Input: part model. Units: mm. Frame: model coordinates. Coordinates: 2 decimals unless noted, no trailing zeros. Write each loop counter-clockwise with the first axis right and the second up, starting at its lowest first coordinate (ties: lowest second). Pieces come first, ordered by that corner, then holes. Notation, with made-up numbers: (17, 28) - (53, 28) arc R20 cw to (53, 60) - close; hole circle Ø11 at (46, 16.5). An arc over 180 degrees is marked (long way). Use CSV: the item, a comma, the result in double quotes.
```python
from build123d import *

# Parameters (mm, degrees)
SKETCH3_R           = 38.1
BOSS_EXTRUDE2_DEPTH = 50.8
SKETCH4_R           = 19.05
FILLET1_R           = 12.7
SKETCH5_R           = 19.05


with BuildPart() as part:
    # Sketch3 → Boss-Extrude2 (new body)
    with BuildSketch(Plane.XY):
        with Locations((0, 177.8)):
            Circle(SKETCH3_R)
    extrude(amount=BOSS_EXTRUDE2_DEPTH)

    # Sweep1: sweep along a curve in space
    with BuildLine() as sweep1_path:
        Line((0, 177.8, 0), (0, 177.8, -76.2))
        Line((0, 177.8, -76.2), (0, 0, -76.2))
        Line((0, 0, -76.2), (0, 0, -177.8))
    # Sketch4 → Sweep1 (sweep)
    with BuildSketch(Plane(origin=(0, 0, 0), x_dir=(-1, 0, 0), z_dir=(0, 0, -1))):
        with Locations((0, 177.8)):
            Circle(SKETCH4_R)
    sweep(path=sweep1_path.line, transition=Transition.RIGHT)

    # Fillet1
    fillet1_edges = [part.edges().sort_by_distance(p)[0] for p in [
        (19.05, 177.8, 0),
    ]]
    fillet(fillet1_edges, radius=FILLET1_R)

    # Sweep2: sweep along a curve in space
    with BuildLine() as sweep2_path:
        Line((0, 0, -177.8), (0, 0, -342.9))
        Line((0, 0, -342.9), (127, 0, -342.9))
        Line((127, 0, -342.9), (127, 0, -469.9))
        Line((127, 0, -469.9), (-12.7, 0, -469.9))
        Line((-12.7, 0, -469.9), (-12.7, 0, -800.1))
        Line((-12.7, 0, -800.1), (102.401088954, 53.669884385, -800.631819274))
        Line((102.401088954, 53.669884385, -800.631819274), (102.401088954, 53.669884385, -927.631819274))
        Line((-12.7, 0, -927.1), (102.401088954, 53.669884385, -927.631819274))
        Line((-12.7, 0, -927.1), (-12.7, 0, -1257.3))
        Line((-12.7, 0, -1257.3), (68.93402643, 97.28289786, -1258.260995676))
        Line((68.93402643, 97.28289786, -1258.260995676), (68.93402643, 97.28289786, -1385.260995676))
        Line((-12.7, 0, -1384.3), (68.93402643, 97.28289786, -1385.260995676))
        Line((-12.7, 0, -1384.3), (-12.7, 0, -1714.5))
        Line((-12.7, 0, -1714.5), (20.170018728, 122.672579939, -1714.5))
        Line((20.170018728, 122.672579939, -1714.5), (20.170018728, 122.672579939, -1841.5))
        Line((-12.7, 0, -1841.5), (20.170018728, 122.672579939, -1841.5))
        Line((-12.7, 0, -1841.5), (-12.7, 0, -2171.7))
        Line((-12.7, 0, -2171.7), (-34.753318564, 125.070584633, -2171.7))
        Line((-34.753318564, 125.070584633, -2171.7), (-34.753318564, 125.070584633, -2298.7))
        Line((-12.7, 0, -2298.7), (-34.753318564, 125.070584633, -2298.7))
        Line((-12.7, 0, -2298.7), (-12.7, 0, -2628.9))
        Line((-12.7, 0, -2628.9), (-85.544207417, 104.032309625, -2628.9))
        Line((-85.544207417, 104.032309625, -2628.9), (-85.544207417, 104.032309625, -2755.9))
        Line((-12.7, 0, -2755.9), (-85.544207417, 104.032309625, -2755.9))
        Line((-12.7, 0, -2755.9), (-12.7, 0, -2895.6))
    # Sketch5 → Sweep2 (sweep)
    with BuildSketch(Plane(origin=(0, 0, -177.8), x_dir=(-1, 0, 0), z_dir=(0, 0, -1))):
        Circle(SKETCH5_R)
    sweep(path=sweep2_path.line, transition=Transition.RIGHT)


solid = part.part
```
(1) Ray query, probe 1 along Z at (x, y) = (-33.5, 94.5); probe 2 along X at (y, z) = (-2, -2333.5); probe 3 along Z at (x, y) = (32, 76.5). Return the intervals inside material, ascending. Write a range as from..to.
Check values:
probe 1,"-2317.31..-2280.09, -2190.31..-2153.09"
probe 2,"-31.64..6.24"
probe 3,"-1396.79..-1373.13, -1269.79..-1246.13"
(2) Pin query (flat end, axial travel): pin 1 Ø6 at (x, z) = (-51.5, -2166.5) entering from +Y; pin 2 Ø12 at (x, y) = (39, 39.5) entering from -Z; pin 3 Ø5 at (x, y) = (19.5, 87.5) entering from +Z. Return the tip coordinate at first contact, or that it passes through.
Check values:
pin 1,"y = 138.26"
pin 2,"z = -1401.97"
pin 3,"z = -67.6"
(3) Draft query along Z for faces 1 (the cylindrical face through (13.928, 59.108, -1377.475)), 2 (the cylindrical face through (0.06, 63.52, -1733.1)), 3 (the cylindrical face through (-4.96, 215.576, 25.044)), 4 (the flat face through (-1, 178, 50.8)). Return one class per face: pulls with the +Z half, pulls with the -Z half, needs draft (parallel to the pull), parting line crosses it, or undercut.
Check values:
face 1,"undercut"
face 2,"undercut"
face 3,"needs draft"
face 4,"pulls with the +Z half"
(4) Cut plane A-A on z = -873.5. Return loops of the section in (x, y).
Check values:
outline,"circle Ø38.1 at (102.4, 53.67)"
